CAD build for the part. Positions are in the model's coordinates, mm. A direction names the side the tool comes from. Give positions to 0.01 mm unless a question says otherwise; leave off trailing zeros. Write each loop counter-clockwise with the first axis right and the second up, starting at its lowest first coordinate (ties: lowest second). Pieces come first, ordered by that corner, then holes. Notation, with made-up numbers: (-24, 55.25) -> (2, 55.25) arc R22 cw to (2, 63.25) -> close; hole circle Ø2 at (-35, -23.5). An arc over 180 degrees is marked (long way). Answer as a JSON object with one key per item and string values.
Autodesk Inventor part; units mm, degrees
ref_plane "Work Plane1" through (-13.4045, 0, 43.75) normal (1, 0, 0) x (0, 1, 0)
ref_plane "Work Plane2" through (-43.75, 0, -26.5955) normal (0, 0, 1) x (0, 1, 0)
ref_plane "YZ Plane" through (0, 0, 0) normal (1, 0, 0) x (0, 1, 0)
sketch "Sketch2" plane through (0, 0, 0) normal (0, 1, 0) x (-1, 0, 0)
  line L0 (-40, -40) -> (40, -40)
  line L1 (40, -40) -> (40, 40)
  line L2 (40, 40) -> (-40, 40)
  line L3 (-40, 40) -> (-40, -40)
  line L4 (-40, -40) -> (40, 40) construction
  line L5 (40, -40) -> (-40, 40) construction
  line L6 (0, 40) -> (40, 40)
  line L7 (20, 40) -> (20, 45)
  line L8 (20, 45) -> (27.5, 45)
  line L9 (20, 40) -> (25, 40)
  line L10 (25, 40) -> (27.5, 45)
  line L11 (20, 45) -> (12.5, 45)
  line L12 (20, 40) -> (15, 40)
  line L13 (15, 40) -> (12.5, 45)
  line L14 (20, 44.75) -> (27.0955, 44.75)
  line L15 (27.0955, 44.75) -> (24.8455, 40.25)
  line L16 (24.8455, 40.25) -> (20, 40.25)
  line L17 (20, 44.75) -> (12.9045, 44.75)
  line L18 (12.9045, 44.75) -> (15.1545, 40.25)
  line L19 (15.1545, 40.25) -> (20, 40.25)
  line L20 (20, 44.75) -> (20, 43.75)
  line L21 (20, 43.75) -> (26.875, 43.75)
  line L22 (20, 43.75) -> (13.125, 43.75)
  line L23 (40, 20) -> (45, 20)
  line L24 (45, 20) -> (45, 27.5)
  line L25 (40, 20) -> (40, 25)
  line L26 (40, 25) -> (45, 27.5)
  line L27 (40, 20) -> (40, 15)
  line L28 (40, 15) -> (45, 12.5)
  line L29 (45, 20) -> (45, 12.5)
  line L30 (44.75, 20) -> (44.75, 27.0955)
  line L31 (44.75, 27.0955) -> (40.25, 24.8455)
  line L32 (40.25, 24.8455) -> (40.25, 20)
  line L33 (44.75, 20) -> (44.75, 12.9045)
  line L34 (44.75, 12.9045) -> (40.25, 15.1545)
  line L35 (40.25, 15.1545) -> (40.25, 20)
  line L36 (44.75, 20) -> (43.75, 20)
  line L37 (43.75, 20) -> (43.75, 26.875)
  line L38 (43.75, 20) -> (43.75, 13.125)
  line L39 (-20, 40) -> (-20, 45)
  line L40 (-20, 44.75) -> (-20, 43.75)
  line L41 (-24.8455, 40.25) -> (-20, 40.25)
  line L42 (-20, 40) -> (-25, 40)
  line L43 (-27.0955, 44.75) -> (-24.8455, 40.25)
  line L44 (-25, 40) -> (-27.5, 45)
  line L45 (-20, 43.75) -> (-26.875, 43.75)
  line L46 (-20, 45) -> (-27.5, 45)
  line L47 (-20, 44.75) -> (-27.0955, 44.75)
  line L48 (-15.1545, 40.25) -> (-20, 40.25)
  line L49 (-20, 40) -> (-15, 40)
  line L50 (-20, 43.75) -> (-13.125, 43.75)
  line L51 (-20, 44.75) -> (-12.9045, 44.75)
  line L52 (-20, 45) -> (-12.5, 45)
  line L53 (-12.9045, 44.75) -> (-15.1545, 40.25)
  line L54 (-15, 40) -> (-12.5, 45)
  line L55 (40, -20) -> (40, -15)
  line L56 (44.75, -12.9045) -> (40.25, -15.1545)
  line L57 (40, -15) -> (45, -12.5)
  line L58 (43.75, -20) -> (43.75, -13.125)
  line L59 (44.75, -20) -> (44.75, -12.9045)
  line L60 (45, -20) -> (45, -12.5)
  line L61 (40.25, -15.1545) -> (40.25, -20)
  line L62 (40, -20) -> (45, -20)
  line L63 (40.25, -24.8455) -> (40.25, -20)
  line L64 (40, -20) -> (40, -25)
  line L65 (44.75, -27.0955) -> (40.25, -24.8455)
  line L66 (40, -25) -> (45, -27.5)
  line L67 (43.75, -20) -> (43.75, -26.875)
  line L68 (44.75, -20) -> (44.75, -27.0955)
  line L69 (45, -20) -> (45, -27.5)
  line L70 (44.75, -20) -> (43.75, -20)
  line L71 (20, -35) -> (27.5, -35)
  line L72 (25, -40) -> (27.5, -35)
  line L73 (20, -35) -> (12.5, -35)
  line L74 (15, -40) -> (12.5, -35)
  line L75 (-15, -40) -> (-12.5, -35)
  line L76 (-20, -35) -> (-12.5, -35)
  line L77 (-25, -40) -> (-27.5, -35)
  line L78 (-20, -35) -> (-27.5, -35)
  line L79 (24.8455, 40.25) -> (24.7205, 40)
  line L80 (15.1545, 40.25) -> (15.2795, 40)
  line L81 (-15.1545, 40.25) -> (-15.2795, 40)
  line L82 (-24.8455, 40.25) -> (-24.7205, 40)
  line L83 (40.25, 24.8455) -> (40, 24.7205)
  line L84 (40.25, 15.1545) -> (40, 15.2795)
  line L85 (40.25, -24.8455) -> (40, -24.7205)
  line L86 (40.25, -15.1545) -> (40, -15.2795)
  line L87 (-40, -25) -> (-35, -27.5)
  line L88 (-35, -20) -> (-35, -27.5)
  line L89 (-35, -20) -> (-35, -12.5)
  line L90 (-40, -15) -> (-35, -12.5)
  line L91 (-35, 20) -> (-35, 12.5)
  line L92 (-35, 20) -> (-35, 27.5)
  line L93 (-40, 15) -> (-35, 12.5)
  line L94 (-40, 25) -> (-35, 27.5)
  point P0 (0, 0)
  point P1 (26.875, -36.25)
  point P2 (13.125, -36.25)
  point P3 (-13.125, -36.25)
  point P4 (-26.875, -36.25)
  point P5 (-13.4045, 43.75)
  point P6 (-26.5955, 43.75)
  point P7 (43.75, -26.5955)
  point P8 (43.75, -13.4045)
  point P9 (43.75, 13.4045)
  point P10 (43.75, 26.5955)
  point P11 (26.5955, 43.75)
  point P12 (13.4045, 43.75)
  point P13 (-36.25, -26.875)
  point P14 (-36.25, -13.125)
  point P15 (-36.25, 13.125)
  point P16 (-36.25, 26.875)
  dimension "d0" = 80
  dimension "d1" = 80
  dimension "d2" = 5
  dimension "d3" = 7.5
  dimension "d4" = 5
  dimension "d5" = 0.25
  dimension "d6" = 0.25
  dimension "d7" = 1
  dimension "d10" = 40
  dimension "d17" = 40
  dimension "d24" = 80
  dimension "d51" = 80
extrude "Extrusion1" add sketch "Sketch2" along normal blind 30 contours L3 L87 L88 L89 L90 L93 L91 L92 L94 L2 L1 L0 L72 L71 L73 L74 L75 L76 L78 L77 | L1 L62 L63 L85 | L82 L41 L39 L2 | L1 L86 L61 L62 | L63 L62 L67 L65 | L39 L48 L81 L2 | L43 L45 L39 L41 | L61 L56 L58 L62 | L39 L50 L53 L48 | L1 L23 L35 L84 | L1 L83 L32 L23 | L35 L23 L38 L34 | L80 L19 L7 L2 | L32 L31 L37 L23 | L7 L16 L79 L2 | L18 L22 L7 L19 | L7 L21 L15 L16
fillet "Fillet1" radius 1 8 edges at (-25, 15, -40) (-15, 15, -40) (15, 15, -40) (25, 15, -40) (40, 15, 15) (40, 15, 25) (40, 15, -15) (40, 15, -25)
fillet "Fillet2" radius 5 4 edges at (-40, 15, 40) (40, 15, 40) (40, 15, -40) (-40, 15, -40)
ref_plane "Work Plane1" through (-13.4045, 0, 43.75) normal (1, 0, 0) x (0, 1, 0)
sketch "Sketch3" plane through (-13.4045, 0, 43.75) normal (1, 0, 0) x (0, 1, 0)
  line L0 (0, -3.75) -> (30, -3.75)
  line L1 (15, -3.75) -> (15, 2)
  line L2 (15, 2) -> (15, 1)
  line L3 (30, -3.75) -> (30, 0)
  arc A0 (30, 0) -> (0, 0) centre (15, -55.25) ccw
  line L4 (30, 0) -> (25, 0)
  line L5 (0, 0) -> (30, 0)
  line L6 (25, 0) -> (5, 0)
  arc A1 (25, 0) -> (5, 0) centre (15, -49.5) ccw
  point P0 (0, -43.75)
  dimension "d34" = 5.75
  dimension "d35" = 1
  dimension "d36" = 5
  dimension "d37" = 20
extrude "Extrusion2" add sketch "Sketch3" against normal blind 13.191 contours L4 A1 L1 A0 | A1 L5 A0 L1
sketch "Sketch4" plane through (0, 30, 0) normal (0, 1, 0) x (1, 0, 0)
  line L0 (-26.5955, -43.75) -> (-13.4045, -43.75)
  line L1 (-20, -43.75) -> (-20, 0)
  line L2 (-20, 0) -> (-43.75, -20)
  line L3 (-43.75, -13.4045) -> (-43.75, -26.5955)
  line L4 (-43.75, -20) -> (-20, -20)
  point P0 (0, 0)
pattern_circular "Circular Pattern1" count 2 over 270 about axis through (-20, 30, 20) along (0, 1, 0) of "Extrusion2"
pattern_linear "Rectangular Pattern1" count 2 spacing 40 along (1, 0, 0) of "Extrusion2"
ref_plane "Work Plane2" through (-43.75, 0, -26.5955) normal (0, 0, 1) x (0, 1, 0)
sketch "Sketch5" plane through (-43.75, 0, -26.5955) normal (0, 0, 1) x (0, 1, 0)
  line L0 (30, 0) -> (30, -3.75)
  line L1 (0, 0) -> (30, 0)
  arc A0 (30, 0) -> (0, 0) centre (15, -55.25) ccw
  arc A1 (25, 0) -> (5, 0) centre (15, -49.5) ccw
  arc A2 (25, 0) -> (5, 0) centre (15, -49.5) ccw
  point P0 (0, -43.75)
extrude "Extrusion3" add sketch "Sketch5" along normal blind 13.191 contours A0 L1 A1
fillet "Fillet3" radius 2 8 edges at (-26.5955, 30, 43.75) (-20, 0, 43.75) (20, 30, 43.75) (20, 0, 43.75) (-43.75, 30, 20) (-43.75, 30, -13.4045) (-43.75, 0, -13.4045) (-43.75, 0, 20)
properties part number "2x2Base"
1) Wall check: probe 1 along Z at (x, y) = (-32, 22.25); probe 2 along Z at (x, y) = (25.5, 16.75). Give the ranges that are in metal, low to high.
Model answer:
{"probe 1": "z = -40 to 40", "probe 2": "z = -35 to 40, 41.56 to 43.75, 44.72 to 45.72"}
2) Slice it at A-A (x = -21.5). List the corners of the cut face in (y, z), then the cut area to 3 significant figures.
Model answer:
{"outline": "(0, -35) -> (30, -35) -> (30, 42.2) arc R2 ccw to (28.47, 44.14) arc R57.25 ccw to (1.53, 44.14) arc R2 ccw to (0, 42.2) -> close; hole (5, 43.75) -> (25, 43.75) arc R50.5 ccw to start", "area": "2,390 mm2"}
3) 3-axis set-ups, long thin cutter, end or side, ignore diameter. For faces 1 (the flat face through (30, 15, 40)), 2 (the cylindrical face through (-45.75, 14.81, -20.09)), 3 (the flat face through (-40, 15, 30)), 4 (the flat face through (-41.9, 14.79, -14.33)), 5 (the flat face through (-25.67, 14.79, 41.9)): which of +Z, -Z, +X, -X, +Y, -Y reach the whole face in a straight line?
Model answer:
{"face 1": "+X, +Y, -Y", "face 2": "+Z, -Z, -X", "face 3": "+Z, +Y, -Y", "face 4": "+Y, -Y", "face 5": "-X, +Y, -Y"}
4) Slice it at C-C (z = -6.5). List the corners of the cut face in (x, y).
Model answer:
{"outline": "(-40, 0) -> (40, 0) -> (40, 30) -> (-40, 30) -> close"}
5) Mould opens along Y. For faces 6 (the flat face through (0, 15, -40)), 7 (the flat face through (20, 15, 43.75)), 8 (the cylindrical face through (20.1, 29.6, 43.4)) say: released by +Y, released by -Y, zero draft, split by the parting line, or undercut.
Model answer:
{"face 6": "zero draft", "face 7": "undercut", "face 8": "released by +Y"}
6) Slice it at B-B (z = -16.5). List the corners of the cut face in (x, y).
Model answer:
{"outline": "(-44.14, 1.53) arc R2 ccw to (-42.2, 0) -> (35, 0) -> (35, 30) -> (-42.2, 30) arc R2 ccw to (-44.14, 28.47) arc R57.25 ccw to start; hole (-43.75, 5) -> (-43.75, 25) arc R50.5 ccw to start"}
7) Slice it at D-D (x = -39). List the corners of the cut face in (y, z), then the cut area to 3 significant figures.
Model answer:
{"outline": "(0, -38) -> (30, -38) -> (30, 38) -> (0, 38) -> close", "area": "2,280 mm2"}
8) Pin check, flat tips, straight feed: pin 1 (16.5 mm diameter, centred on x = 20.5, y = 22, fed in from -Z); pin 2 (1 mm diameter, centred on y = 9, z = 45, fed in from -X); pin 3 (1.6 mm diameter, centred on x = -44.5, y = 11, fed in from -Z); pin 4 (6.5 mm diameter, centred on x = 19, y = 10, fed in from +Z). Stop position of each tip, or through.
Model answer:
{"pin 1": "stops at z = -40", "pin 2": "stops at x = -26.6", "pin 3": "stops at z = -26.6", "pin 4": "stops at z = 45.72"}
